Geometry: final body of the model. Coordinates: model frame, mm. Give positions to 0.01 mm unless a question says otherwise; leave off trailing zeros. Write each loop counter-clockwise with the first axis right and the second up, starting at its lowest first coordinate (ties: lowest second). Pieces come first, ordered by that corner, then holes. Notation, with made-up numbers: (-4.75, -27.75) -> (42.25, -27.75) arc R12 cw to (42.25, -21.75) -> close; hole circle Ø10 at (89, 53.5). An arc over 180 degrees is marked (long way). Answer in a Markdown table with one row per item. Add a question column.
Item 1: First-contact query: P1, Ø3, axis at x = 22.5, y = 20.5, coming from the -Z side; P2, Ø12, axis at x = 27, y = -20, coming from the -Z side. Flat tips, straight axial feed; report the tip coordinate or a pass-through.
Item 2: Section query C-C on z = 1.75. Output: boundary loops of the cut face in (x, y), plus the area to 3 significant figures.
Item 3: Section query D-D on x = -15. Output: boundary loops of the cut face in (y, z), plus the area to 3 significant figures.
Item 4: Section query B-B on x = 0. Output: boundary loops of the cut face in (y, z), plus the area to 3 significant figures.
Item 5: Draft query along Y for faces 1 (the cylindrical face through (0.504, 48.075, 2.535)), 2 (the flat face through (-35, -7, 2)), 3 (the cylindrical face through (21.026, 21.852, 2.535)), 4 (the flat face through (0, -52.5, 2)). Return one class per face: +Y half, -Y half, draft (parallel to the pull), parting line (faces both ways), or undercut.
Item 6: Section query A-A on y = 20.5. Output: boundary loops of the cut face in (x, z).
Item 7: Material intervals for probe 1 along Y at (x, z) = (0, 1.45); probe 2 along Y at (x, z) = (21.5, 0.8); probe 3 along X at (y, z) = (22, 3.8), sorted ascending. Write a range as from..to.
```python
from build123d import *

# Parameters (mm, degrees)
SKETCH1_W           = 70
SKETCH1_H           = 105
BOSS_EXTRUDE1_DEPTH = 5
SKETCH2_R           = 17.5
CUT_EXTRUDE3_DEPTH  = 64.294944506
SKETCH3_R           = 2
CUT_EXTRUDE4_DEPTH  = 64.294944506
SKETCH4_R           = 2
CUT_EXTRUDE5_DEPTH  = 5
CUT_EXTRUDE6_DEPTH  = 10


with BuildPart() as part:
    # Sketch1 → Boss-Extrude1 (new body)
    with BuildSketch(Plane.XY):
        Rectangle(SKETCH1_W, SKETCH1_H)
    extrude(amount=BOSS_EXTRUDE1_DEPTH)

    # Sketch2 → Cut-Extrude3 (cut, through all)
    with BuildSketch(Plane(origin=(0, 0, 0), x_dir=(-1, 0, 0), z_dir=(0, 0, -1))):
        with Locations((0, 20.5)):
            Circle(SKETCH2_R)
    extrude(amount=-CUT_EXTRUDE3_DEPTH, mode=Mode.SUBTRACT)

    # Sketch3 → Cut-Extrude4 (cut, through all)
    with BuildSketch(Plane.XY.offset(5)):
        with Locations((-22.5, 20.5)):
            Circle(SKETCH3_R)
        with Locations((0, 43)):
            Circle(SKETCH3_R)
        with Locations((22.5, 20.5)):
            Circle(SKETCH3_R)
    extrude(amount=-CUT_EXTRUDE4_DEPTH, mode=Mode.SUBTRACT)

    # Sketch4 → Cut-Extrude5 (cut)
    with BuildSketch(Plane.XY.offset(5)):
        with Locations((0, -42.5)):
            Circle(SKETCH4_R)
        with Locations((-23, -17.5)):
            Circle(SKETCH4_R)
        with Locations(Location((23, -17.5, 0), (0, 0, 180))):
            Circle(SKETCH4_R)
    extrude(amount=-CUT_EXTRUDE5_DEPTH, mode=Mode.SUBTRACT)

    # Sketch5 → Cut-Extrude6 (cut)
    with BuildSketch(Plane.XY.offset(5)):
        with BuildLine():
            Line((-35, 40.793543502), (-35, 52.5))
            Line((-35, 52.5), (35, 52.5))
            Line((35, 52.5), (35, 40.793543502))
            ThreePointArc((35, 40.793543502), (0, 48.07644174), (-35, 40.793543502))
        make_face()
    extrude(amount=-CUT_EXTRUDE6_DEPTH, mode=Mode.SUBTRACT)


solid = part.part
```
Findings below:
| question | item | result |
|---|---|---|
| 1 | P1 | passes through |
| 1 | P2 | stops at z = 0 |
| 2 | outline | (-35, -52.5) -> (35, -52.5) -> (35, 40.79) arc R87.74 ccw to (-35, 40.79) -> close; hole circle Ø4 at (-23, -17.5); hole circle Ø4 at (-22.5, 20.5); hole circle Ø35 at (0, 20.5); hole circle Ø4 at (0, -42.5); hole circle Ø4 at (0, 43); hole circle Ø4 at (22.5, 20.5); hole circle Ø4 at (23, -17.5) |
| 2 | area | 5,840 mm^2 |
| 3 | outline | (-52.5, 0) -> (11.49, 0) -> (11.49, 5) -> (-52.5, 5) -> close; (29.51, 0) -> (46.78, 0) -> (46.78, 5) -> (29.51, 5) -> close |
| 3 | area | 406 mm^2 |
| 4 | outline | (-52.5, 0) -> (-44.5, 0) -> (-44.5, 5) -> (-52.5, 5) -> close; (-40.5, 0) -> (3, 0) -> (3, 5) -> (-40.5, 5) -> close; (38, 0) -> (41, 0) -> (41, 5) -> (38, 5) -> close; (45, 0) -> (48.08, 0) -> (48.08, 5) -> (45, 5) -> close |
| 4 | area | 288 mm^2 |
| 5 | face 1 | +Y half |
| 5 | face 2 | draft |
| 5 | face 3 | undercut |
| 5 | face 4 | -Y half |
| 6 | outline | (-35, 0) -> (-24.5, 0) -> (-24.5, 5) -> (-35, 5) -> close; (-20.5, 0) -> (-17.5, 0) -> (-17.5, 5) -> (-20.5, 5) -> close; (17.5, 0) -> (20.5, 0) -> (20.5, 5) -> (17.5, 5) -> close; (24.5, 0) -> (35, 0) -> (35, 5) -> (24.5, 5) -> close |
| 7 | probe 1 | y = -52.5..-44.5, -40.5..3, 38..41, 45..48.08 |
| 7 | probe 2 | y = -52.5..-18.82, -16.18..18.77, 22.23..45.4 |
| 7 | probe 3 | x = -35..-23.82, -21.18..-17.44, 17.44..21.18, 23.82..35 |
